Can you work these out from the model? Positions are in its coordinate system, mm. Give positions to 0.01 mm unless a question says otherwise; leave off trailing zeros. Write each loop counter-clockwise with the first axis right and the second up, starting at its lowest first coordinate (ties: lowest second). Pieces come first, ordered by that corner, then holes. Notation, with made-up numbers: M 76.25,4.25 L 90.25,4.25 A26 cw 90.25,29.25 Z; hole C 22.25,20 d8. An arc over 180 degrees is marked long. Use CSV: the item, a comma, the result in double quotes. Start each with the question number.
from build123d import *

# Parameters (mm, degrees)
SKETCH_1_W           = 2.54
SKETCH_1_H           = 2.54
EXTRUDE_1_DEPTH      = 2.54
EXTRUDE_2_DEPTH      = 8.03
EXTRUDE_2_DEPTH_BACK = 1.73
SKETCH_2_W           = 0.64
SKETCH_2_H           = 0.64
SKETCH_3_W           = 0.46
SKETCH_3_H           = 0.46
EXTRUDE_3_DEPTH      = 0.51
SKETCH_4_W           = 0.46
SKETCH_4_H           = 0.46
EXTRUDE_4_DEPTH      = 0.51
DRAFT_2_ANGLE        = 10
DRAFT_3_ANGLE        = 10
CHAMFER_1_SIZE       = 0.509116882


with BuildPart() as part:
    # ｽｹｯﾁ1 → ﾎﾞｽ - 押し出し1 (new body)
    with BuildSketch(Plane.XY):
        Rectangle(SKETCH_1_W, SKETCH_1_H)
    extrude(amount=EXTRUDE_1_DEPTH)

    # ｽｹｯﾁ2 → ﾎﾞｽ - 押し出し2 (add, two sides: drawn at the far end of the back side and taken through both)
    with BuildSketch(Plane.XY.offset(-EXTRUDE_2_DEPTH_BACK)):
        Rectangle(SKETCH_2_W, SKETCH_2_H)
    extrude(amount=EXTRUDE_2_DEPTH + EXTRUDE_2_DEPTH_BACK)

    # ｽｹｯﾁ3 → ﾎﾞｽ - 押し出し3 (add)
    with BuildSketch(Plane(origin=(0, 0, -1.73), x_dir=(-1, 0, 0), z_dir=(0, 0, -1))):
        Rectangle(SKETCH_3_W, SKETCH_3_H)
    extrude(amount=EXTRUDE_3_DEPTH)

    # ｽｹｯﾁ4 → ﾎﾞｽ - 押し出し4 (add)
    with BuildSketch(Plane.XY.offset(8.03)):
        Rectangle(SKETCH_4_W, SKETCH_4_H)
    extrude(amount=EXTRUDE_4_DEPTH)

    # 抜き勾配2
    draft_2_faces = [part.faces().sort_by_distance(p)[0] for p in [
        (0, -0.23, 8.285),
        (-0.23, 0, 8.285),
        (0, 0.23, 8.285),
        (0.23, 0, 8.285),
    ]]
    draft(draft_2_faces, Plane.XY.offset(8.54), DRAFT_2_ANGLE)

    # 抜き勾配3
    draft_3_faces = [part.faces().sort_by_distance(p)[0] for p in [
        (-0.23, 0, -1.985),
        (0, -0.23, -1.985),
        (0.23, 0, -1.985),
        (0, 0.23, -1.985),
    ]]
    draft(draft_3_faces, Plane(origin=(0, 0, -2.24), x_dir=(-1, 0, 0), z_dir=(0, 0, -1)), DRAFT_3_ANGLE)

    # 面取り1
    chamfer_1_edges = [part.edges().sort_by_distance(p)[0] for p in [
        (1.27, -1.27, 1.27),
        (-1.27, -1.27, 1.27),
        (-1.27, 1.27, 1.27),
        (1.27, 1.27, 1.27),
    ]]
    chamfer(chamfer_1_edges, length=CHAMFER_1_SIZE)


solid = part.part
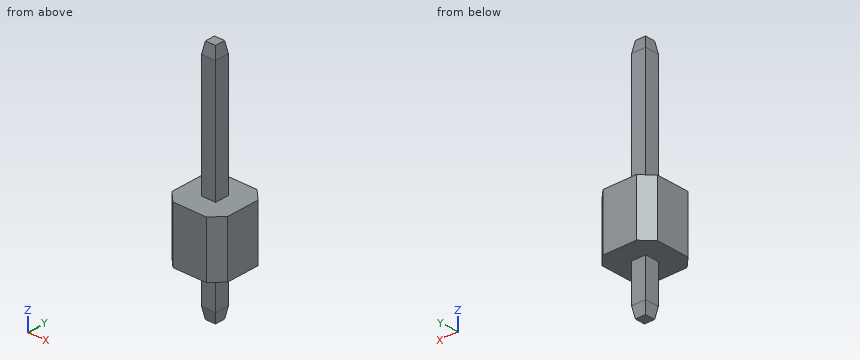
(1) Please list where these lines run through material, in increasing order: L1, parallel to Y at x = -0.1, z = 7; L2, parallel to Z at x = 0.55, y = -0.15. Write a range as [from, to].
(2) Will these pins go through, and if not, where does the flat tip stop? pin 1 Ø0.7 at (x, z) = (0, 5) entering from -Y; pin 2 Ø0.5 at (x, z) = (0, -1) entering from +Y; pin 3 Ø0.5 at (y, z) = (0, 6) entering from -X.
(3) I want a section at B-B (z = 2.25). Write out the boundary of the cut face in (x, y).
(4) I want a section at D-D (y = -0.45). Write out the boundary of the cut face in (x, z), and give its area (3 significant figures).
Geometry results:
1,L1,"y = [-0.32, 0.32]"
1,L2,"z = [0, 2.54]"
2,pin 1,"stops at y = -0.32"
2,pin 2,"stops at y = 0.32"
2,pin 3,"stops at x = -0.32"
3,outline,"M -1.27,-0.76 L -0.76,-1.27 L 0.76,-1.27 L 1.27,-0.76 L 1.27,0.76 L 0.76,1.27 L -0.76,1.27 L -1.27,0.76 Z"
4,outline,"M -1.27,0 L 1.27,0 L 1.27,2.54 L -1.27,2.54 Z"
4,area,"6.45 mm2"
